Answer from the drawing. Dimensions are ordinates in mm from the lowest x, y and z of the part. Round coordinates to 2 decimals unless told otherwise and drop trailing zeros. Order: outer loops, then holes, each group sorted by start corner. A loop starts at its lowest first (then second) coordinate and runs counter-clockwise, first axis right, second up. Notation, with made-up numbers: M 8,65.25 L 49,65.25 A20 cw 49,79.25 Z; hole C 78,88 d4. An arc over 180 degrees is marked long. Answer as a JSON object with one key per item and string values. Group by question number.
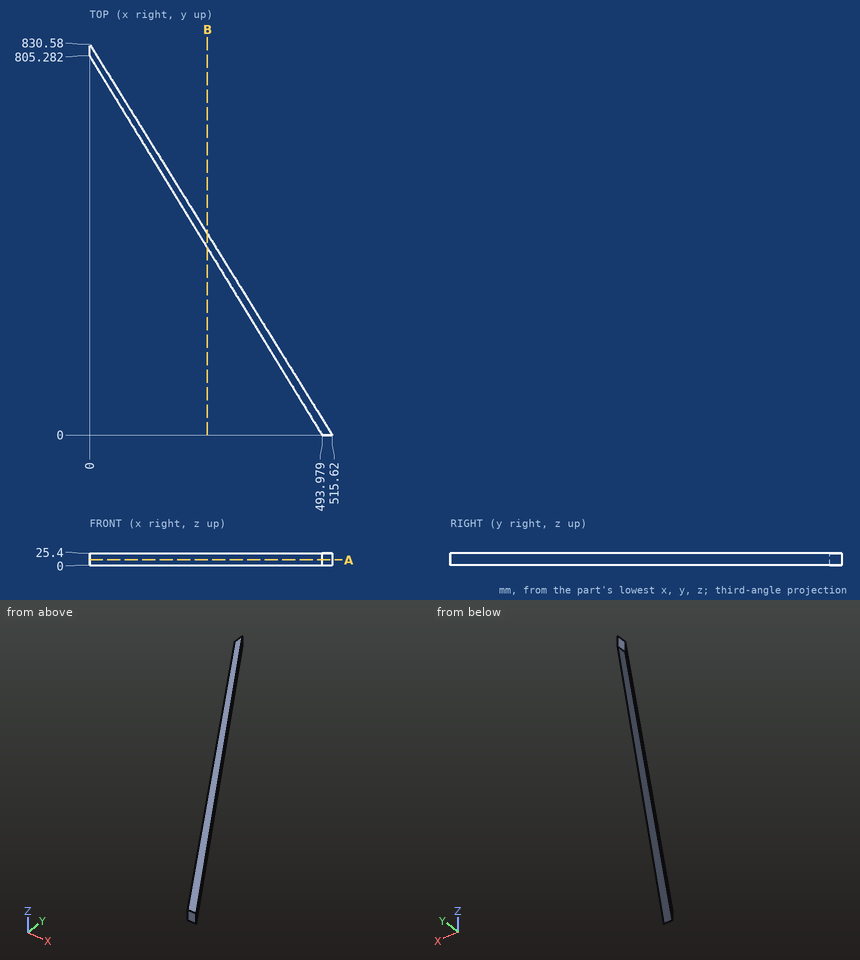
Item 1: Find section B-B (x = 250.5). Give the vertices of the cut face in (y, z) (1 decimal), and give its area (3 significant figures).
Item 2: Each of these flat-tipped pins is pushed along its axis until it touches: pin 1 (8 mm diameter, centred on x = 439, z = 12, fed in from +Y) (1 decimal); pin 2 (1.5 mm diameter, centred on y = 581.5, z = 22.5, fed in from +X); pin 3 (5 mm diameter, centred on y = 169, z = 2.5, fed in from +X). Where does it stop, or does it pass through?
Item 3: Consider L1, parallel to Y at x = 447, z = 3.5 (1 decimal); L2, parallel to Y at x = 87, z = 5.75 (1 decimal); L3, parallel to X at y = 288, z = 22.75. Determine where each line is inside the solid, lowest interval first.
Item 4: Find section A-A (z = 11.25). Give the vertices of the cut face in (x, y), and give its area (3 significant figures).
Responses:
{
 "1": {"outline": "M 396.9,0 L 427.1,0 L 427.1,25.4 L 396.9,25.4 Z", "area": "766 mm^2"},
 "2": {"pin 1": "stops at y = 129.9", "pin 2": "stops at x = 155.09", "pin 3": "stops at x = 412.26"},
 "3": {"L1": "y = 76.6 to 110.5", "L2": "y = 663.5 to 690.4", "L3": "x = 317.31 to 336.83"},
 "4": {"outline": "M 0,805.28 L 493.98,0 L 515.62,0 L 0,830.58 Z", "area": "15,200 mm^2"}
}
